Autodesk Inventor part; units mm, degrees
ref_plane "YZ Plane" through (0, 0, 0) normal (1, 0, 0) x (0, 1, 0)
ref_plane "XZ Plane" through (0, 0, 0) normal (0, 1, 0) x (-1, 0, 0)
ref_plane "XY Plane" through (0, 0, 0) normal (0, 0, 1) x (1, 0, 0)
sketch "Sketch1" plane through (0, 0, 0) normal (0, 0, 1) x (1, 0, 0)
  line L0 (0, 0) -> (30.734, 0)
  line L1 (30.734, 0) -> (30.734, -106.934)
  line L2 (30.734, -106.934) -> (0, -106.934)
  line L3 (0, -106.934) -> (0, 0)
  dimension "d0" = 30.734
  dimension "d1" = 106.934
extrude "Extrusion1" add sketch "Sketch1" along normal blind 10
fillet "Fillet1" radius 3.175 4 edges at (0, 0, 5) (30.734, 0, 5) (30.734, -106.934, 5) (0, -106.934, 5)
sketch "Sketch2" plane through (30.734, -103.759, 0) normal (1, 0, 0) x (0, 0, -1)
  line L0 (-7.5, 26.825) -> (-2.5, 26.825)
  line L1 (-2.5, 26.825) -> (-2.5, 38.825)
  line L2 (-2.5, 38.825) -> (-7.5, 38.825)
  line L3 (-7.5, 38.825) -> (-7.5, 26.825)
  line L4 (-10, -3.175) -> (0, -3.175)
  line L5 (-10, -3.175) -> (-10, 0)
  line L6 (-7.5, 46.825) -> (-2.5, 46.825)
  line L7 (-2.5, 46.825) -> (-2.5, 58.825)
  line L8 (-2.5, 58.825) -> (-7.5, 58.825)
  line L9 (-7.5, 58.825) -> (-7.5, 46.825)
  line L10 (-7.5, 66.825) -> (-2.5, 66.825)
  line L11 (-2.5, 66.825) -> (-2.5, 78.825)
  line L12 (-2.5, 78.825) -> (-7.5, 78.825)
  line L13 (-7.5, 78.825) -> (-7.5, 66.825)
  line L14 (-7.5, 86.825) -> (-2.5, 86.825)
  line L15 (-2.5, 86.825) -> (-2.5, 98.825)
  line L16 (-2.5, 98.825) -> (-7.5, 98.825)
  line L17 (-7.5, 98.825) -> (-7.5, 86.825)
  point P0 (0, 103.759)
  point P1 (-5, 26.825)
  point P2 (-5, -3.175)
  point P3 (-5, 46.825)
  point P4 (-5, 66.825)
  point P5 (-5, 86.825)
  dimension "d5" = 30
  dimension "d6" = 12
  dimension "d7" = 5
  dimension "d10" = 20
extrude "Extrusion2" cut sketch "Sketch2" against normal blind 10
sketch "Sketch3" plane through (30.734, -103.759, 0) normal (1, 0, 0) x (0, 0, -1)
  line L0 (-6.5, 17.825) -> (-3.5, 17.825)
  line L1 (-3.5, 17.825) -> (-3.5, 18.825)
  line L2 (-3.5, 18.825) -> (-6.5, 18.825)
  line L3 (-6.5, 18.825) -> (-6.5, 17.825)
  line L4 (-10, -3.175) -> (0, -3.175)
  point P0 (0, 103.759)
  point P1 (-5, 17.825)
  point P2 (-5, -3.175)
  dimension "d17" = 21
  dimension "d18" = 1
  dimension "d19" = 3
extrude "Extrusion3" cut sketch "Sketch3" against normal blind 0.1
sketch "Sketch4" plane through (20.734, -103.759, 0) normal (1, 0, 0) x (0, 0, -1)
  line L0 (-6.5, 27.825) -> (-5.5, 27.825)
  line L1 (-5.5, 27.825) -> (-5.5, 37.825)
  line L2 (-5.5, 37.825) -> (-6.5, 37.825)
  line L3 (-6.5, 37.825) -> (-6.5, 27.825)
  line L4 (-7.5, 26.825) -> (-7.5, 38.825)
  line L5 (-2.5, 26.825) -> (-7.5, 26.825)
  line L6 (-7.5, 38.825) -> (-2.5, 38.825)
  line L7 (-6.5, 47.825) -> (-5.5, 47.825)
  line L8 (-5.5, 47.825) -> (-5.5, 57.825)
  line L9 (-5.5, 57.825) -> (-6.5, 57.825)
  line L10 (-6.5, 57.825) -> (-6.5, 47.825)
  line L11 (-6.5, 67.825) -> (-5.5, 67.825)
  line L12 (-5.5, 67.825) -> (-5.5, 77.825)
  line L13 (-5.5, 77.825) -> (-6.5, 77.825)
  line L14 (-6.5, 77.825) -> (-6.5, 67.825)
  line L15 (-6.5, 87.825) -> (-5.5, 87.825)
  line L16 (-5.5, 87.825) -> (-5.5, 97.825)
  line L17 (-5.5, 97.825) -> (-6.5, 97.825)
  line L18 (-6.5, 97.825) -> (-6.5, 87.825)
  point P0 (0, 103.759)
  point P1 (-6.5, 32.825)
  point P2 (-7.5, 32.825)
  point P3 (-6.5, 52.825)
  point P4 (-6.5, 72.825)
  point P5 (-6.5, 92.825)
  dimension "d24" = 1
  dimension "d25" = 1
  dimension "d26" = 1
  dimension "d29" = 20
extrude "Extrusion4" add sketch "Sketch4" along normal blind 8
sketch "Sketch5" plane through (3.175, -106.934, 0) normal (0, -1, 0) x (1, 0, 0)
  line L0 (9.192, 9) -> (15.192, 9)
  line L1 (15.192, 9) -> (15.192, 1)
  line L2 (15.192, 1) -> (9.192, 1)
  line L3 (9.192, 1) -> (9.192, 9)
  line L4 (0, 10) -> (24.384, 10)
  line L5 (24.384, 0) -> (0, 0)
  point P0 (-3.175, 0)
  point P1 (12.192, 9)
  point P2 (12.192, 10)
  dimension "d36" = 6
  dimension "d37" = 1
  dimension "d38" = 1
extrude "Extrusion5" cut sketch "Sketch5" against normal blind 5
sketch "Sketch6" plane through (12.367, -106.934, 1) normal (0, 0, 1) x (1, 0, 0)
  line L0 (6, 0) -> (0, 0)
  line L1 (6, 0) -> (6, 5)
  line L2 (6, 5) -> (0, 5)
  line L3 (0, 0) -> (0, 5)
  line L4 (-9, 0) -> (15, 0)
  line L5 (-9, 0) -> (0, 5)
  line L6 (15.192, 0) -> (-9.192, 0)
  line L7 (6, 5) -> (15.192, 0)
  point P0 (-12.367, 106.934)
  point P1 (3, 0)
  dimension "d41" = 24
extrude "Extrusion6" cut sketch "Sketch6" along normal blind 8 contours L1 L7 L6 L4 | L4 L5 L3
properties part number "USB Hub" material "ABS Plastic"
Input: part model. Units: mm. Frame: model coordinates. A direction names the side the tool comes from. Round coordinates to 2 decimals unless told otherwise and drop trailing zeros. Loops run counter-clockwise (first coordinate to the right, second up) from the corner with the lowest first, then second, coordinate; pieces in that order, holes last.
1) Pull-direction query (Z, two-part tool) for faces 4 (the flat face through (15, -53, 10)), 5 (the flat face through (25, -51, 5.5)), 6 (the cylindrical face through (0.905, -105.979, 5.07)), 7 (the flat face through (26, -31, 2.5)); classes: released by +Z, released by -Z, zero draft, split by the parting line, or undercut.
Ans:
face 4: released by +Z
face 5: undercut
face 6: zero draft
face 7: undercut
2) Section query C-C on x = 16. Return the cut outline in (y, z).
Ans:
outline: (-106.93, 0) - (0, 0) - (0, 10) - (-106.93, 10) - (-106.93, 9) - (-101.93, 9) - (-101.93, 1) - (-106.93, 1) - close
3) Pin query (flat end, axial travel): pin 1 (1.1 mm diameter, centred on y = -31, z = 6, fed in from +X); pin 2 (0.5 mm diameter, centred on y = -85.5, z = 4.5, fed in from +X); pin 3 (1.5 mm diameter, centred on y = -11.5, z = 4.5, fed in from +X). Return the tip coordinate at first contact, or that it passes through.
Ans:
pin 1: stops at x = 28.73
pin 2: stops at x = 30.63
pin 3: stops at x = 20.73
4) Material intervals for line 1 (Z direction, x = 22, y = -34); line 2 (Z direction, x = 28, y = -65); line 3 (X direction, y = -65, z = 5.75), sorted ascending.
Ans:
line 1: z = 0 to 2.5, 5.5 to 6.5, 7.5 to 10
line 2: z = 0 to 2.5, 7.5 to 10
line 3: x = 0 to 20.73
5) Section query D-D on x = 7. Return the cut outline in (y, z), plus the area to 3 significant figures.
Ans:
outline: (-106.93, 0) - (0, 0) - (0, 10) - (-106.93, 10) - (-106.93, 9) - (-104.92, 9) - (-104.92, 1) - (-106.93, 1) - close
area: 1,050 mm2
6) Set-up query: faces 1 (the flat face through (15, -101.934, 5)), 2 (the flat face through (25, -31, 5.5)), 3 (the cylindrical face through (29.829, -0.955, 5.07)). Return all of +Z, -Z, +X, -X, +Y, -Y with unobstructed straight access to the full face (end or side cutting, diameter ignored); none if empty.
Ans:
face 1: -Y
face 2: +X
face 3: +Z, -Z, +X, +Y
7) Section query A-A on y = -9.5. Return the cut outline in (x, z), plus the area to 3 significant figures.
Ans:
outline: (0, 0) - (30.73, 0) - (30.73, 2.5) - (20.73, 2.5) - (20.73, 5.5) - (28.73, 5.5) - (28.73, 6.5) - (20.73, 6.5) - (20.73, 7.5) - (30.73, 7.5) - (30.73, 10) - (0, 10) - close
area: 265 mm2
